Input: part model. Units: mm. Frame: model coordinates. Give positions to 0.01 mm unless a question says otherwise; leave off trailing zeros. Loops run counter-clockwise (first coordinate to the right, second up) from the corner with the lowest first, then second, coordinate; pieces in that order, holes last. Notation, with made-up numbers: M 78,8 L 114,8 A36 ccw 114,43 Z; hole C 69,62.5 d7. An arc over 180 degrees is marked long. Use CSV: the item, a comma, the result in double quotes. Start each with the question number.
Q1. Section B-B, the plane z = 2.75. State how many separate pieces and enclosed holes the cut face has, plus the area to 3 significant figures.
Q2. Section D-D, the plane y = 155. Output: boundary loops of the cut face in (x, z) (3 decimals), plus the area to 3 significant figures.
Q3. Pin query (flat end, axial travel): pin 1 (5 mm diameter, centred on x = 45, y = 115, fed in from +Z); pin 2 (8 mm diameter, centred on x = 122, z = 3.5, fed in from +Y). Return the tip coordinate at first contact, or that it passes through.
Q4. Section C-C, the plane x = 88. Output: boundary loops of the cut face in (y, z), plus the area to 3 significant figures.
Q5. Material intervals for line 1 along Y through (x, z) = (15, 6.75); line 2 along X through (y, z) = (85, 8.25); line 3 along X through (y, z) = (185, 9) (3 decimals), sorted ascending.
Q6. Section A-A, the plane y = 85. Output: boundary loops of the cut face in (x, z).
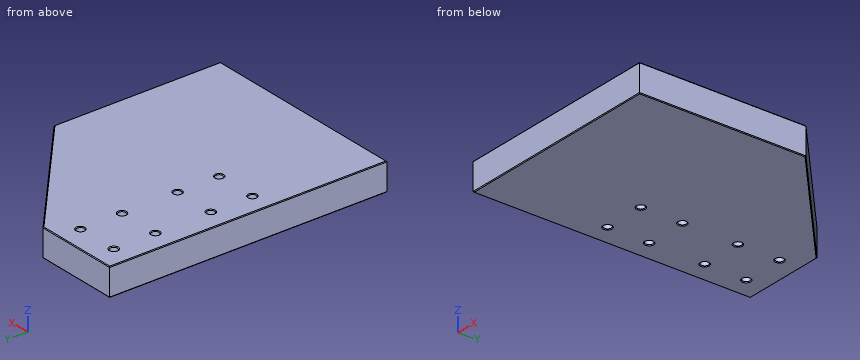
Autodesk Inventor part; units mm, degrees
ref_plane "YZ Plane" through (0, 0, 0) normal (1, 0, 0) x (0, 1, 0)
ref_plane "XZ Plane" through (0, 0, 0) normal (0, 1, 0) x (-1, 0, 0)
ref_plane "XY Plane" through (0, 0, 0) normal (0, 0, 1) x (1, 0, 0)
sketch "Skizze1" plane through (0, 0, 0) normal (0, 0, 1) x (1, 0, 0)
  line L0 (0, 0) -> (0, 200)
  line L1 (0, 200) -> (60, 200)
  line L2 (0, 0) -> (150, 0)
  line L3 (150, 0) -> (150, 120)
  line L4 (150, 120) -> (60, 200)
  dimension "d0" = 200
  dimension "d1" = 60
  dimension "d2" = 150
  dimension "d3" = 120
extrude "Extrusion1" add sketch "Skizze1" along normal blind 20
sketch "Skizze2" plane through (0, 0, 20) normal (0, 0, 1) x (1, 0, 0)
  line L0 (60, 200) -> (0, 200)
  line L1 (30, 200) -> (30, 170) construction
  line L2 (30, 170) -> (30, 100) construction
  line L3 (15, 155) -> (45, 155) construction
  line L4 (45, 155) -> (45, 185) construction
  line L5 (45, 185) -> (15, 185) construction
  line L6 (15, 185) -> (15, 155) construction
  line L7 (15, 155) -> (45, 185) construction
  line L8 (45, 155) -> (15, 185) construction
  line L9 (15, 85) -> (45, 85) construction
  line L10 (45, 85) -> (45, 115) construction
  line L11 (45, 115) -> (15, 115) construction
  line L12 (15, 115) -> (15, 85) construction
  line L13 (15, 85) -> (45, 115) construction
  line L14 (45, 85) -> (15, 115) construction
  point P0 (0, 0)
  dimension "d6" = 30
  dimension "d7" = 70
  dimension "d8" = 30
  dimension "d9" = 30
  dimension "d10" = 30
  dimension "d11" = 30
hole "Bohrung1" at (15, 185, 20) at (45, 185, 20) at (15, 155, 20) at (45, 155, 20) at (15, 115, 20) at (45, 115, 20) at (15, 85, 20) at (45, 85, 20) direction (0, 0, -1) diameter 5.5 end through all
chamfer "Fase1" distance 0.5 angle 45 18 edges at (30, 200, 20) (105, 160, 20) (150, 60, 20) (75, 0, 20) (0, 100, 20) (15, 87.75, 20) (15, 117.75, 20) (45, 87.75, 20) (45, 117.75, 20) (15, 157.75, 20) (15, 187.75, 20) (45, 157.75, 20) (45, 187.75, 20) (105, 160, 0) (30, 200, 0) (0, 100, 0) (150, 60, 0) (75, 0, 0)
chamfer "Fase2" distance 0.5 angle 45 8 edges at (15, 87.75, 0) (15, 117.75, 0) (45, 87.75, 0) (45, 117.75, 0) (15, 157.75, 0) (15, 187.75, 0) (45, 157.75, 0) (45, 187.75, 0)
properties part number "Portalwange" material "Aluminium 6061"
A:
1,separate pieces,"1"
1,enclosed holes,"8"
1,area,"26,200 mm^2"
2,outline,"M 0,0.5 L 0.5,0 L 11.75,0 L 12.25,0.5 L 12.25,19.5 L 11.75,20 L 0.5,20 L 0,19.5 Z; M 17.75,0.5 L 18.25,0 L 41.75,0 L 42.25,0.5 L 42.25,19.5 L 41.75,20 L 18.25,20 L 17.75,19.5 Z; M 47.75,0.5 L 48.25,0 L 109.872,0 L 110.625,0.5 L 110.625,19.5 L 109.872,20 L 48.25,20 L 47.75,19.5 Z"
2,area,"1,990 mm^2"
3,pin 1,"through"
3,pin 2,"y = 148.44"
4,outline,"M 0,0.5 L 0.5,0 L 174.44,0 L 175.11,0.5 L 175.11,19.5 L 174.44,20 L 0.5,20 L 0,19.5 Z"
4,area,"3,500 mm^2"
5,line 1,"0 to 82.25, 87.75 to 112.25, 117.75 to 152.25, 157.75 to 182.25, 187.75 to 200"
5,line 2,"0 to 12.25, 17.75 to 42.25, 47.75 to 150"
5,line 3,"0 to 12.25, 17.75 to 42.25, 47.75 to 76.875"
6,outline,"M 0,0.5 L 0.5,0 L 11.75,0 L 12.25,0.5 L 12.25,19.5 L 11.75,20 L 0.5,20 L 0,19.5 Z; M 17.75,0.5 L 18.25,0 L 41.75,0 L 42.25,0.5 L 42.25,19.5 L 41.75,20 L 18.25,20 L 17.75,19.5 Z; M 47.75,0.5 L 48.25,0 L 149.5,0 L 150,0.5 L 150,19.5 L 149.5,20 L 48.25,20 L 47.75,19.5 Z"
